Build history of the part. All positions in model axes, mm. Give positions to 0.01 mm unless a question says otherwise; leave off trailing zeros. Write each loop counter-clockwise with the first axis right and the second up, starting at its lowest first coordinate (ties: lowest second). Pieces come first, ordered by that corner, then holes. Notation, with made-up numbers: M 82,11 L 120,11 A22 cw 120,34 Z; hole C -8.75,7 d10. An arc over 180 degrees is marked long. Return JSON: item names as keys, results as strings. Group by question number.
Q1. Band-saw the part on C-C, the plane z = 254. Give the cut face in (x, y), then the cut area to 3 significant figures.
Q2. Band-saw the part on B-B, the plane y = -73.5. Give the cut face in (x, z), then the cut area to 3 significant figures.
Q3. Band-saw the part on A-A, the plane y = 19. Give the cut face in (x, z).
Q4. Band-saw the part on D-D, the plane z = -129. Give the cut face in (x, y), then the cut area to 3 significant figures.
Q5. Wall check: probe 1 along Z at (x, y) = (-15.5, 19); probe 2 along Z at (x, y) = (-15, -74); probe 3 along Z at (x, y) = (-16, 19). Give the ranges that are in metal, low to high.
Q6. Flat gauge pins, fed straight in: pin 1 Ø9 at (x, z) = (-20, 259.5) entering from -Y; pin 2 Ø6 at (x, y) = (-23.5, -95) entering from +Z; pin 3 Ø11.5 at (y, z) = (19, 254) entering from -X. Where does each tip first touch, or does it go through?
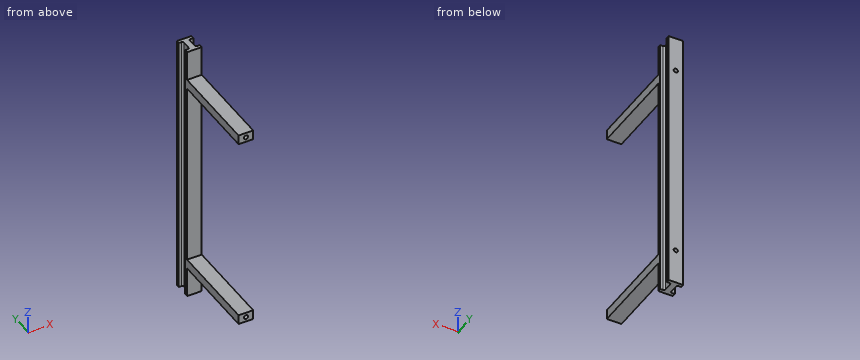
Autodesk Inventor part; units mm, degrees
ref_plane "YZ Plane" through (0, 0, 0) normal (1, 0, 0) x (0, 1, 0)
ref_plane "XZ Plane" through (0, 0, 0) normal (0, 1, 0) x (-1, 0, 0)
ref_plane "XY Plane" through (0, 0, 0) normal (0, 0, 1) x (1, 0, 0)
sketch "Sketch1" plane through (0, 0, 0) normal (0, 0, 1) x (1, 0, 0)
  line L0 (0, 0) -> (-30.5, 0)
  line L1 (-30.5, 0) -> (-30.5, 38)
  line L2 (-30.5, 38) -> (0, 38)
  line L3 (0, 38) -> (0, 0)
  line L4 (0, 0) -> (0, 7)
  line L5 (0, 38) -> (0, 31)
  line L6 (0, 31) -> (-6, 31)
  line L7 (0, 7) -> (-6, 7)
  line L8 (-9, 10) -> (-9, 28)
  line L9 (-30.5, 38) -> (-30.5, 31)
  line L10 (-30.5, 31) -> (-24.5, 31)
  line L11 (-21.5, 28) -> (-21.5, 10)
  line L12 (-30.5, 0) -> (-30.5, 7)
  line L13 (-30.5, 7) -> (-24.5, 7)
  arc A0 (-6, 31) -> (-9, 28) centre (-6, 28) ccw
  arc A1 (-9, 10) -> (-6, 7) centre (-6, 10) ccw
  arc A2 (-21.5, 28) -> (-24.5, 31) centre (-24.5, 28) ccw
  arc A3 (-24.5, 7) -> (-21.5, 10) centre (-24.5, 10) ccw
  point P0 (-9, 31)
  point P1 (-21.5, 31)
  dimension "d0" = 30.5
  dimension "d1" = 38
  dimension "d2" = 7
  dimension "d3" = 7
  dimension "d4" = 9
  dimension "d6" = 7
  dimension "d7" = 9
  dimension "d8" = 7
  dimension "d9" = 3
  dimension "d11" = 3
extrude "Extrusion1" add sketch "Sketch1" along normal mid plane 558.8 contours L0 L1 L13 A3 L11 A2 L10 L2 L3 L6 A0 L8 A1 L7
hole "Hole1" at (-9, 19, 254) direction (-1, 0, 0) diameter 10 depth 25
sketch "Sketch7" plane through (-9, 10, 279.4) normal (1, 0, 0) x (0, 0, -1)
  line L0 (558.8, 18) -> (558.8, 0)
  line L1 (558.8, 18) -> (0, 18)
  point P0 (533.4, 9)
  dimension "d23" = 25.4
  dimension "d25" = 9
hole "Hole2" at (-9, 19, -254) direction (-1, 0, 0) diameter 10 depth 25 tip angle 118
sketch "Sketch2" plane through (-30.5, 0, 279.4) normal (0, -1, 0) x (1, 0, 0)
  line L0 (0, 0) -> (30.5, 0)
  line L1 (15.25, 0) -> (15.25, -63.5)
  line L2 (15.25, -63.5) -> (0, -63.5)
  line L3 (0, -558.8) -> (0, 0)
  line L4 (15.25, -63.5) -> (30.5, -63.5)
  line L5 (30.5, -63.5) -> (30.5, -83.5)
  line L6 (30.5, -558.8) -> (30.5, 0)
  line L7 (30.5, -83.5) -> (0, -83.5)
  line L8 (0, -83.5) -> (0, -63.5)
  line L9 (30.5, -558.8) -> (0, -558.8)
  line L10 (15.25, -558.8) -> (15.25, -495.3)
  line L11 (15.25, -495.3) -> (30.5, -495.3)
  line L12 (15.25, -495.3) -> (0, -495.3)
  line L13 (0, -495.3) -> (0, -475.3)
  line L14 (0, -475.3) -> (30.5, -475.3)
  line L15 (30.5, -475.3) -> (30.5, -495.3)
  point P0 (30.5, -279.4)
  dimension "d33" = 63.5
  dimension "d34" = 20
  dimension "d35" = 30.5
  dimension "d36" = 63.5
  dimension "d37" = 20
extrude "Extrusion2" add sketch "Sketch2" along normal blind 190 contours L2 L4 L5 L7 L3 | L14 L6 L11 L12 L3
sketch "Sketch5" plane through (-30.5, 38, 279.4) normal (0, 1, 0) x (1, 0, 0)
  point P0 (30.5, 279.4)
sketch "Sketch10" plane through (-30.5, -190, 279.4) normal (0, -1, 0) x (1, 0, 0)
  line L0 (30.5, -495.3) -> (30.5, -475.3)
  line L1 (0, -495.3) -> (30.5, -495.3)
  point P0 (30.5, -279.4)
  point P1 (15.5, -485.3)
  dimension "d82" = 15
  dimension "d83" = 10
hole "Hole6" at (-15, -190, -205.9) direction (0, 1, 0) diameter 8.647 end through all
sketch "Sketch11" plane through (-30.5, -190, 279.4) normal (0, -1, 0) x (1, 0, 0)
  line L0 (30.5, -83.5) -> (30.5, -63.5)
  line L1 (0, -83.5) -> (30.5, -83.5)
  point P0 (30.5, -279.4)
  point P1 (15.5, -73.5)
  dimension "d91" = 15
  dimension "d92" = 10
hole "Hole7" at (-15, -190, 205.9) direction (0, 1, 0) diameter 8.647 end through all
properties part number "Barra"
From the geometry:
{
 "1": {"outline": "M -30.5,0 L 0,0 L 0,7 L -6,7 A3 cw -9,10 L -9,14 L -21.5,14 L -21.5,10 A3 cw -24.5,7 L -30.5,7 Z; M -30.5,31 L -24.5,31 A3 cw -21.5,28 L -21.5,24 L -9,24 L -9,28 A3 cw -6,31 L 0,31 L 0,38 L -30.5,38 Z", "area": "610 mm^2"},
 "2": {"outline": "M -30.5,-215.9 L 0,-215.9 L 0,-195.9 L -30.5,-195.9 Z; M -30.5,195.9 L 0,195.9 L 0,215.9 L -30.5,215.9 Z; hole C -15,-205.9 d8.65; hole C -15,205.9 d8.65", "area": "1,100 mm^2"},
 "3": {"outline": "M -21.5,-279.4 L -9,-279.4 L -9,-259 L -21.5,-259 Z; M -21.5,-249 L -9,-249 L -9,249 L -21.5,249 Z; M -21.5,259 L -9,259 L -9,279.4 L -21.5,279.4 Z; hole C -15,-205.9 d8.65; hole C -15,205.9 d8.65"},
 "4": {"outline": "M -30.5,0 L 0,0 L 0,7 L -6,7 A3 cw -9,10 L -9,28 A3 cw -6,31 L 0,31 L 0,38 L -30.5,38 L -30.5,31 L -24.5,31 A3 cw -21.5,28 L -21.5,10 A3 cw -24.5,7 L -30.5,7 Z", "area": "735 mm^2"},
 "5": {"probe 1": "z = -279.4 to -259, -249 to -210.19, -201.61 to 201.61, 210.19 to 249, 259 to 279.4", "probe 2": "z = -215.9 to -210.22, -201.58 to -195.9, 195.9 to 201.58, 210.22 to 215.9", "probe 3": "z = -279.4 to -259, -249 to -210.11, -201.69 to 201.69, 210.11 to 249, 259 to 279.4"},
 "6": {"pin 1": "stops at y = 0", "pin 2": "stops at z = 215.9", "pin 3": "stops at x = -21.5"}
}
